```python
from build123d import *

# Parameters (mm, degrees)
SKETCH1_R             = 82.5
BOSS_EXTRUDE1_DEPTH   = 22
SKETCH2_R             = 27.5
CUT_EXTRUDE1_DEPTH    = 119.728682297
SKETCH3_R             = 2.473860502
CUT_EXTRUDE2_DEPTH    = 18.704156
CIRPATTERN1_START     = 3.295843645
CIRPATTERN1_OUTLINE_R = 2.473860502
CIRPATTERN1_DEPTH     = 18.704156355


# Read off the part's stored shape, not the designer's step: CirPattern1
with BuildPart() as part:
    # Sketch1 → Boss-Extrude1 (new body)
    with BuildSketch(Plane(origin=(0, 0, 0), x_dir=(1, 0, 0), z_dir=(0, 1, 0))):
        with Locations(Location((0, 0, 0), (0, 0, 270))):
            Circle(SKETCH1_R)
    extrude(amount=BOSS_EXTRUDE1_DEPTH)

    # Sketch2 → Cut-Extrude1 (cut, through all)
    with BuildSketch(Plane(origin=(0, 0, 0), x_dir=(1, 0, 0), z_dir=(0, 1, 0))):
        with Locations(Location((0, 0, 0), (0, 0, 270))):
            Circle(SKETCH2_R)
    extrude(amount=CUT_EXTRUDE1_DEPTH, mode=Mode.SUBTRACT)

    # Sketch3 → Cut-Extrude2 (cut)
    with BuildSketch(Plane(origin=(0, 22, 0), x_dir=(1, 0, 0), z_dir=(0, 1, 0))):
        with Locations(Location((-37.202802875, 0, 0), (0, 0, 270))):
            Circle(SKETCH3_R)
    extrude(amount=-CUT_EXTRUDE2_DEPTH, mode=Mode.SUBTRACT)

    # CirPattern1 outline → CirPattern1 (cut)
    with BuildSketch(Plane(origin=(0, 0, 0), x_dir=(1, 0, 0), z_dir=(0, 1, 0)).offset(CIRPATTERN1_START)):
        with Locations((-26.306354192, -26.306354192)):
            Circle(CIRPATTERN1_OUTLINE_R)
        with Locations((-26.306354192, 26.306354192)):
            Circle(CIRPATTERN1_OUTLINE_R)
        with Locations((0, 37.202802875)):
            Circle(CIRPATTERN1_OUTLINE_R)
        with Locations((26.306354192, 26.306354192)):
            Circle(CIRPATTERN1_OUTLINE_R)
        with Locations((37.202802875, 0)):
            Circle(CIRPATTERN1_OUTLINE_R)
        with Locations((26.306354192, -26.306354192)):
            Circle(CIRPATTERN1_OUTLINE_R)
        with Locations((0, -37.202802875)):
            Circle(CIRPATTERN1_OUTLINE_R)
    extrude(amount=CIRPATTERN1_DEPTH, mode=Mode.SUBTRACT)


solid = part.part
```
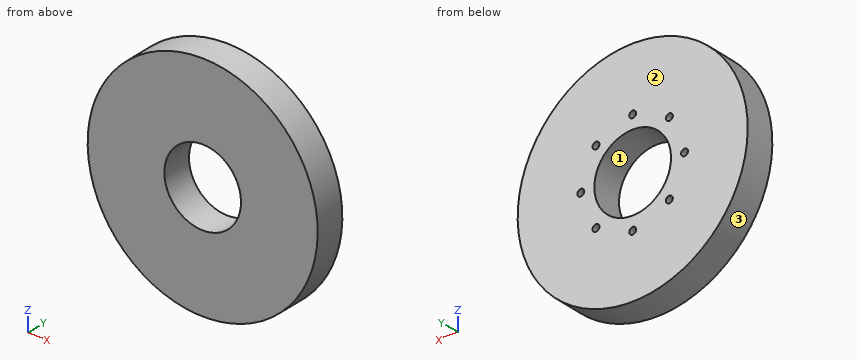
Work out the finished part from the listing and answer in its coordinate system (mm). Face numbers are marked on the shaded views. Round coordinates to 2 decimals unless told otherwise and drop trailing zeros. Loops run counter-clockwise (first coordinate to the right, second up) from the corner with the lowest first, then second, coordinate; pieces in that order, holes last. Notation, with made-up numbers: (-39, 27) -> (2, 27) arc R26 cw to (2, 50) -> close; hole circle Ø3 at (85, 69.25). An arc over 180 degrees is marked (long way). Write each question's results on one line, items separated by ' | '. Start each with the question number.
1. Find the intervals of material crossed by probe 1 along X at (y, z) = (15.25, 0); probe 2 along X at (y, z) = (19.5, -22.5); probe 3 along Z at (x, y) = (18, 9.5), in increasing order. Write a range as from..to.
2. Section C-C (y = 10.25) is taken. State how many separate pieces and enclosed holes the cut face has, plus the area to 3 significant figures.
3. Given pin 1 Ø4.5 at (x, z) = (26.31, -26.31) entering from +Y; pin 2 Ø4 at (y, z) = (17.5, 36.5) entering from -X; pin 3 Ø3 at (y, z) = (3.5, 41.5) entering from -X, each flat-ended and moving along its own axis, determine where each tip first touches the part or whether it passes through.
4. Section A-A (x = 0) is taken. Determine the outline of the cut face in (y, z).
5. For a pull along X with two mould halves and no side action, classify the marked faces 1, 2 and 3 as +X half, -X half, draft (parallel to the pull), parting line (faces both ways), or undercut.
6. Section D-D (z = -19.5) is taken. Determine the outline of the cut face in (x, y), plus the area to 3 significant figures.
7. Section B-B (z = 0) is taken. Determine the outline of the cut face in (x, y).
Evaluation:
1) probe 1: x = -82.5..-39.68, -34.73..-27.5, 27.5..34.73, 39.68..82.5 | probe 2: x = -79.37..-15.81, 15.81..79.37 | probe 3: z = -80.51..-20.79, 20.79..80.51
2) separate pieces: 1 | enclosed holes: 9 | area: 18,900 mm2
3) pin 1: stops at y = 3.3 | pin 2: stops at x = -74.94 | pin 3: stops at x = -72.15
4) outline: (0, -82.5) -> (22, -82.5) -> (22, -39.68) -> (3.3, -39.68) -> (3.3, -34.73) -> (22, -34.73) -> (22, -27.5) -> (0, -27.5) -> close; (0, 27.5) -> (22, 27.5) -> (22, 34.73) -> (3.3, 34.73) -> (3.3, 39.68) -> (22, 39.68) -> (22, 82.5) -> (0, 82.5) -> close
5) face 1: undercut | face 2: draft | face 3: parting line
6) outline: (-80.16, 0) -> (-19.39, 0) -> (-19.39, 22) -> (-80.16, 22) -> close; (19.39, 0) -> (80.16, 0) -> (80.16, 22) -> (19.39, 22) -> close | area: 2,670 mm2
7) outline: (-82.5, 0) -> (-27.5, 0) -> (-27.5, 22) -> (-34.73, 22) -> (-34.73, 3.3) -> (-39.68, 3.3) -> (-39.68, 22) -> (-82.5, 22) -> close; (27.5, 0) -> (82.5, 0) -> (82.5, 22) -> (39.68, 22) -> (39.68, 3.3) -> (34.73, 3.3) -> (34.73, 22) -> (27.5, 22) -> close
